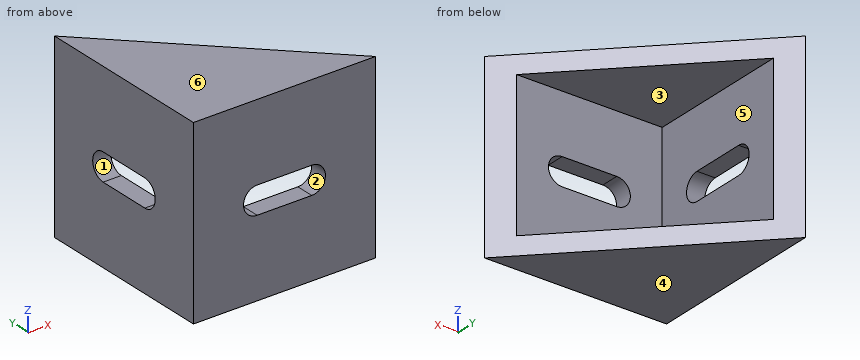
```python
from build123d import *

# Parameters (mm, degrees)
BOSS_EXTRUDE1_DEPTH = 20
SHELL1_T            = -2
CUT_EXTRUDE1_DEPTH  = 20
CUT_EXTRUDE2_DEPTH  = 20


with BuildPart() as part:
    # Sketch1 → Boss-Extrude1 (new body)
    with BuildSketch(Plane.XY):
        Polygon((-10, 10), (10, -10), (-10, -10), align=None)
    extrude(amount=BOSS_EXTRUDE1_DEPTH)

    # Shell1
    shell1_openings = [part.faces().sort_by_distance(p)[0] for p in [
        (0, 0, 10),
    ]]
    offset(amount=SHELL1_T, openings=shell1_openings, kind=Kind.INTERSECTION)

    # Sketch2 → Cut-Extrude1 (cut)
    with BuildSketch(Plane(origin=(-8, 0, 0), x_dir=(0, 0, -1), z_dir=(1, 0, 0))):
        with BuildLine():
            Line((-11.5, 3), (-11.5, -3))
            ThreePointArc((-11.5, -3), (-10, -4.5), (-8.5, -3))
            Line((-8.5, -3), (-8.5, 3))
            ThreePointArc((-8.5, 3), (-10, 4.5), (-11.5, 3))
        make_face()
    extrude(amount=-CUT_EXTRUDE1_DEPTH, mode=Mode.SUBTRACT)

    # Sketch3 → Cut-Extrude2 (cut)
    with BuildSketch(Plane(origin=(0, -8, 0), x_dir=(1, 0, 0), z_dir=(0, 1, 0))):
        with BuildLine():
            Line((-3, -8.5), (3, -8.5))
            ThreePointArc((3, -8.5), (4.5, -10), (3, -11.5))
            Line((3, -11.5), (-3, -11.5))
            ThreePointArc((-3, -11.5), (-4.5, -10), (-3, -8.5))
        make_face()
    extrude(amount=-CUT_EXTRUDE2_DEPTH, mode=Mode.SUBTRACT)


solid = part.part
```
Source: CAD feature listing. Evaluate the final solid. Frame: model axes, mm. Face numbers are marked on the shaded views. A direction names the side the tool comes from. Round coordinates to 2 decimals unless told otherwise and drop trailing zeros. Loops run counter-clockwise (first coordinate to the right, second up) from the corner with the lowest first, then second, coordinate; pieces in that order, holes last.
(1) Contact query for flat-ended pins moving along their axis: pin 1 Ø1 at (y, z) = (-3.5, 18) entering from +X; pin 2 Ø8 at (y, z) = (4, 10) entering from +X. Output: stop coordinate, or through.
From the geometry:
pin 1: stops at x = 4
pin 2: stops at x = -8
(2) Access query for the marked faces 1, 2 and 3. Directions: +Z, -Z, +X, -X, +Y, -Y. A direction counts if a zero-diameter tool reaches every point of the face in a straight line with its end or side. Return the directions, or none.
From the geometry:
face 1: +X, -X
face 2: +Y, -Y
face 3: +X, +Y
(3) Pull-direction query (Z, two-part tool) for the marked faces 4, 5 and 6; classes: +Z half, -Z half, draft (parallel to the pull), parting line (faces both ways), or undercut.
From the geometry:
face 4: -Z half
face 5: undercut
face 6: +Z half
(4) Section query B-B (z = 10). Output: boundary loops of the cut face in (x, y), and give its area (3 significant figures).
From the geometry:
outline: (-10, -10) - (-4.5, -10) - (-4.5, -8) - (-8, -8) - (-8, -4.5) - (-10, -4.5) - close; (-10, 4.5) - (-8, 4.5) - (-8, 8) - (-10, 10) - close; (4.5, -10) - (10, -10) - (8, -8) - (4.5, -8) - close
area: 36.0 mm2
(5) Section query C-C (x = 0). Output: boundary loops of the cut face in (y, z).
From the geometry:
outline: (-10, 0) - (0, 0) - (0, 2) - (-8, 2) - (-8, 8.5) - (-10, 8.5) - close; (-10, 11.5) - (-8, 11.5) - (-8, 18) - (0, 18) - (0, 20) - (-10, 20) - close
(6) Material intervals for probe 1 along Z at (x, y) = (-6, 5); probe 2 along Z at (x, y) = (-9, 0.5); probe 3 along X at (y, z) = (6.25, 14), sorted ascending.
From the geometry:
probe 1: z = 0 to 2, 18 to 20
probe 2: z = 0 to 8.5, 11.5 to 20
probe 3: x = -10 to -8
(7) Section query D-D (x = 7.25). Output: boundary loops of the cut face in (y, z).
From the geometry:
outline: (-10, 0) - (-7.25, 0) - (-7.25, 2) - (-8, 2) - (-8, 18) - (-7.25, 18) - (-7.25, 20) - (-10, 20) - close
(8) Section query A-A (y = 2.5). Output: boundary loops of the cut face in (x, z), and give its area (3 significant figures).
From the geometry:
outline: (-10, 0) - (-2.5, 0) - (-2.5, 2) - (-8, 2) - (-8, 8.5) - (-10, 8.5) - close; (-10, 11.5) - (-8, 11.5) - (-8, 18) - (-2.5, 18) - (-2.5, 20) - (-10, 20) - close
area: 56.0 mm2
